```python
from build123d import *

# Parameters (mm, degrees)
F0_W     = 6.4
F0_H     = 5
F1_DEPTH = 3.3
F2_R     = 1
F3_R     = 0.5
F4_DEPTH = 5.001


with BuildPart() as f1:
    # F0 (on Top) → F1 (new body)
    with BuildSketch(Plane.XY):
        with Locations((3.2, 2.5)):
            Rectangle(F0_W, F0_H)
    extrude(amount=F1_DEPTH)

    # F2
    f2_edges = [f1.edges().sort_by_distance(p)[0] for p in [
        (0, 2.5, 3.3),
        (6.4, 2.5, 3.3),
        (6.4, 2.5, 0),
        (0, 2.5, 0),
    ]]
    fillet(f2_edges, radius=F2_R)

    # F3 (on face) → F4 (cut, through all)
    with BuildSketch(Plane.XZ):
        with Locations((1.5, 1.65)):
            Circle(F3_R)
        with Locations((4.9, 1.65)):
            Circle(F3_R)
    extrude(amount=-F4_DEPTH, mode=Mode.SUBTRACT)


solid = f1.part
```
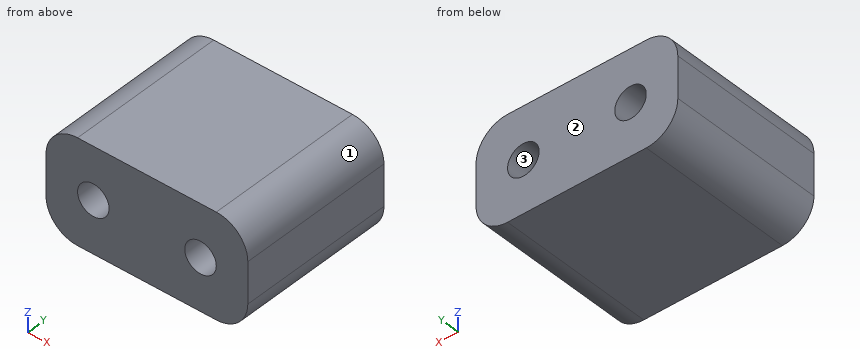
CAD build for the part. Positions are in the model's coordinates, mm. Face numbers are marked on the shaded views. Round coordinates to 2 decimals unless told otherwise and drop trailing zeros. Order: outer loops, then holes, each group sorted by start corner. A loop starts at its lowest first (then second) coordinate and runs counter-clockwise, first axis right, second up.
Item 1: Mould opens along Z. For the marked faces 1, 2 and 3 say: pulls with the +Z half, pulls with the -Z half, needs draft (parallel to the pull), parting line crosses it, or undercut.
Item 2: Saw through at B-B on x = 1.5. Write the cut outline in (y, z), then the cut area to 3 significant figures.
Item 3: Saw through at D-D on z = 0.6. Write the cut outline in (x, y).
Item 4: Saw through at A-A on z = 1.65. Write the cut outline in (x, y), then the cut area to 3 significant figures.
Item 5: Saw through at C-C on y = 3.5. Write the cut outline in (x, z).
Item 6: Probe line 1 along Z through (x, y) = (4.9, 3.35); line 2 along X through (y, z) = (3.2, 1.5); line 3 along X through (y, z) = (4.25, 1.95). List the from-to ranges inside material, lowest first.
Reported:
1. face 1: pulls with the +Z half
1. face 2: needs draft
1. face 3: undercut
2. outline: (0, 0) - (5, 0) - (5, 1.15) - (0, 1.15) - close; (0, 2.15) - (5, 2.15) - (5, 3.3) - (0, 3.3) - close
2. area: 11.5 mm2
3. outline: (0.08, 0) - (6.32, 0) - (6.32, 5) - (0.08, 5) - close
4. outline: (0, 0) - (1, 0) - (1, 5) - (0, 5) - close; (2, 0) - (4.4, 0) - (4.4, 5) - (2, 5) - close; (5.4, 0) - (6.4, 0) - (6.4, 5) - (5.4, 5) - close
4. area: 22.0 mm2
5. outline: (0, 1) arc R1 ccw to (1, 0) - (5.4, 0) arc R1 ccw to (6.4, 1) - (6.4, 2.3) arc R1 ccw to (5.4, 3.3) - (1, 3.3) arc R1 ccw to (0, 2.3) - close; hole circle Ø1 at (1.5, 1.65); hole circle Ø1 at (4.9, 1.65)
6. line 1: z = 0 to 1.15, 2.15 to 3.3
6. line 2: x = 0 to 1.02, 1.98 to 4.42, 5.38 to 6.4
6. line 3: x = 0 to 1.1, 1.9 to 4.5, 5.3 to 6.4
